Job drawing, mm, ordinate dimensions from the low corner. One solid piece. A direction names the side the tool comes from. Give positions to 0.01 mm unless a question says otherwise; leave off trailing zeros. Order: outer loops, then holes, each group sorted by start corner. A loop starts at its lowest first (then second) coordinate and runs counter-clockwise, first axis right, second up. Notation, with made-up numbers: M 70,61 L 119,61 A14 ccw 119,65 Z; hole C 36.25,8.25 d6. An arc over 180 degrees is marked long. Put each result on its own line as item: value. Start each with the question number.
1) Cut at D-D (z = 12). Write the cut outline in (x, y).
2) Drill centre lines: line 1 (X direction, y = 40, z = 41); line 2 (Z direction, x = 57, y = 37.5); line 3 (Y direction, x = 15, z = 5). Where is each one in solid material? Low to high. Write a range as [from, to].
3) Tool access for the marked faces 1, 2 and 3: list every direction of +Z, -Z, +X, -X, +Y, -Y with a clear straight run to the whole face (end or side of a thin tool).
4) Cut at B-B (x = 41.5). Write the cut outline in (y, z), and give its area (3 significant figures).
5) Cut at A-A (z = 22.5). Write the cut outline in (x, y).
6) Cut at C-C (y = 38.5). Write the cut outline in (x, z).
7) Pin check, flat tips, straight feed: pin 1 (6 mm diameter, centred on x = 61.5, z = 8, fed in from -Y); pin 2 (16 mm diameter, centred on y = 36, z = 45, fed in from -X); pin 3 (8 mm diameter, centred on x = 11, z = 24.5, fed in from +Y); pin 4 (13.5 mm diameter, centred on x = 42, y = 27, fed in from -Z). Stop position of each tip, or through.
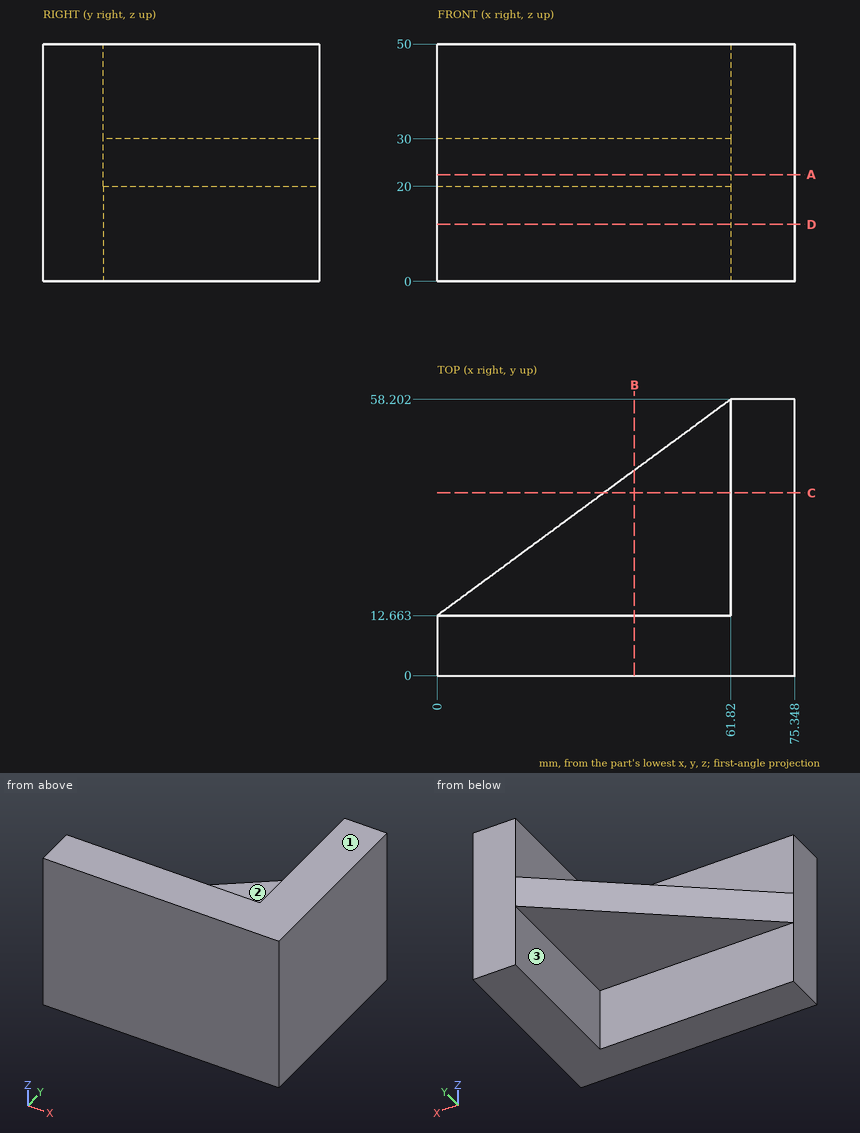
Solution:
1. outline: M 0,0 L 75.35,0 L 75.35,58.2 L 61.82,58.2 L 61.82,12.66 L 0,12.66 Z
2. line 1: [61.82, 75.35]
2. line 2: [20, 30]
2. line 3: [0, 12.66]
3. face 1: +Z, +X, -X, +Y, -Y
3. face 2: +Z, -X, +Y
3. face 3: -Z, -X, +Y
4. outline: M 0,0 L 12.66,0 L 12.66,20 L 43.23,20 L 43.23,30 L 12.66,30 L 12.66,50 L 0,50 Z
4. area: 939 mm²
5. outline: M 0,0 L 75.35,0 L 75.35,58.2 L 61.82,58.2 L 0,12.66 Z
6. outline: M 35.07,20 L 61.82,20 L 61.82,0 L 75.35,0 L 75.35,50 L 61.82,50 L 61.82,30 L 35.07,30 Z
7. pin 1: y = 0
7. pin 2: x = 61.82
7. pin 3: y = 23.71
7. pin 4: z = 20
